```python
from build123d import *

# Parameters (mm, degrees)
F0_W     = 400
F0_H     = 200
F1_DEPTH = 5
F2_R     = 7.5
F3_DEPTH = 25
F5_R     = 7.5
F6_DEPTH = 25


with BuildPart() as f1:
    # F0 (on Top) → F1 (new body)
    with BuildSketch(Plane.XY):
        with Locations((0.230974, 4.11826)):
            Rectangle(F0_W, F0_H)
    extrude(amount=F1_DEPTH)


with BuildPart() as f3:
    # F2 (on Top) → F3 (new body)
    with BuildSketch(Plane.XY):
        with Locations((121.673325, 0)):
            Circle(F2_R)
    extrude(amount=F3_DEPTH)


with BuildPart() as f1_1:
    add(f1.part)

    # F4: cut F3
    add(f3.part, mode=Mode.SUBTRACT)


with BuildPart() as f6:
    # F5 (on Top) → F6 (new body)
    with BuildSketch(Plane.XY):
        with Locations((-117.027458, 0)):
            Circle(F5_R)
    extrude(amount=F6_DEPTH)


with BuildPart() as f1_2:
    add(f1_1.part)

    # F7: cut F6
    add(f6.part, mode=Mode.SUBTRACT)


solid = f1_2.part
```
Here's how the part is built. I have some questions about the finished solid (model axes, mm). Give positions to 0.01 mm unless a question says otherwise; leave off trailing zeros. Write each loop counter-clockwise with the first axis right and the second up, starting at its lowest first coordinate (ties: lowest second). Pieces come first, ordered by that corner, then holes.
(1) Thinking about a two-plate mould opening in X: for faces 1 (the face through (-109.874, 2.253, 2.465)), 2 (the face through (-3, 6, 5)), which applies, pulls with the +X half, pulls with the -X half, needs draft (parallel to the pull), parting line crosses it, or undercut?
Output values:
face 1: undercut
face 2: needs draft
(2) Imagine slicing it at A-A, the plane y = 0. Write out the boundary of the cut face in (x, z).
Output values:
outline: (-199.77, 0) - (-124.53, 0) - (-124.53, 5) - (-199.77, 5) - close; (-109.53, 0) - (114.17, 0) - (114.17, 5) - (-109.53, 5) - close; (129.17, 0) - (200.23, 0) - (200.23, 5) - (129.17, 5) - close
(3) Will this pin go through, and if not, where does the flat tip stop? pin 1 (12 mm diameter, centred on x = 121.67, y = 0, fed in from +Z).
Output values:
pin 1: passes through
(4) If I drill on L1, parallel to X at y = 0, z = 3.95, over which ranges is the centre line in solid material (lowest first)?
Output values:
L1: x = -199.77 to -124.53, -109.53 to 114.17, 129.17 to 200.23
(5) Imagine slicing it at B-B, the plane x = 118. Write out the boundary of the cut face in (y, z).
Output values:
outline: (-95.88, 0) - (-6.54, 0) - (-6.54, 5) - (-95.88, 5) - close; (6.54, 0) - (104.12, 0) - (104.12, 5) - (6.54, 5) - close
